from build123d import *

# Parameters (mm, degrees)
F1_DEPTH  = 8
F3_W      = 8
F3_H      = 8
F3_R      = 2.4
F4_DEPTH  = 1.7
F5_R      = 2.4
F6_DEPTH  = 1.7
F11_W     = 31.0510899872
F11_H     = 25.4
F12_DEPTH = 7.9248


with BuildPart() as f1:
    # F0 (on Front) → F1 (new body)
    with BuildSketch(Plane.XZ):
        Polygon((-2.4, 9.6), (-4, 9.6), (-4, 0), (4, 0), (4, 9.6), (2.4, 9.6), (2.4, 11.3), (-2.4, 11.3), align=None)
    extrude(amount=F1_DEPTH)

    # F3 (on plane+point) → F4 (cut, through all)
    with BuildSketch(Plane.XY.offset(11.3)):
        with Locations((0, -4)):
            Rectangle(F3_W, F3_H)
        with Locations((0, -4)):
            Circle(F3_R, mode=Mode.SUBTRACT)
    extrude(amount=-F4_DEPTH, mode=Mode.SUBTRACT)

    # F5 (on Top) → F6 (cut)
    with BuildSketch(Plane.XY):
        with Locations((0, -4)):
            Circle(F5_R)
    extrude(amount=F6_DEPTH, mode=Mode.SUBTRACT)

    # F8: F1 across plane


with BuildPart() as f1_1:
    add(f1.part)
    add(f1.part.mirror(Plane.YZ.offset(4)))

    # F9: F1 across face


with BuildPart() as f1_2:
    add(f1_1.part)
    add(f1_1.part.mirror(Plane(origin=(4, -8, 4.8), x_dir=(1, 0, 0), z_dir=(0, -1, 0))))

    # F10: F1 across face


with BuildPart() as f1_3:
    add(f1_2.part)
    add(f1_2.part.mirror(Plane(origin=(4, -16, 4.8), x_dir=(1, 0, 0), z_dir=(0, -1, 0))))

    # F11 (on Front) → F12 (cut)
    with BuildSketch(Plane.XZ):
        with Locations((3.3294046298, 0)):
            Rectangle(F11_W, F11_H)
    extrude(amount=F12_DEPTH, mode=Mode.SUBTRACT)


solid = f1_3.part
Could you check a few things on this model? Use its own coordinates, in mm. A direction names the side the tool comes from. Round coordinates to 2 decimals unless told otherwise and drop trailing zeros. Write each loop counter-clockwise with the first axis right and the second up, starting at its lowest first coordinate (ties: lowest second). Pieces come first, ordered by that corner, then holes. Notation, with made-up numbers: (-5.75, -16) - (26.25, -16) arc R24 cw to (26.25, -6) - close; hole circle Ø10 at (17, 79.5). An arc over 180 degrees is marked (long way). Put each result on its own line as item: value. Start each with the question number.
(1) I want a section at C-C, the plane y = -29.5. Please give me the cut outline in (x, z), plus the area to 3 significant figures.
(2) Will this pin go through, and if not, where does the flat tip stop? pin 1 (2 mm diameter, centred on x = 8, y = -11.5, fed in from -Z).
(3) For faces 1 (the flat face through (4, -20, 0)), 2 (the cylindrical face through (8.52, -22.343, 10.462)), 3 (the flat face through (8, -20, 1.7)), which set-ups out of +Z, -Z, +X, -X, +Y, -Y let a thin tool reach every point of the face, with its end or its side?
(4) Thinking about a two-plate mould opening in Y: for faces 4 (the flat face through (12, -20, 5)), 5 (the flat face through (8, -28, 1.7)), 6 (the flat face through (4, -7.925, 5)), 7 (the cylindrical face through (8.52, -22.343, 0.838)), which applies, released by +Y, released by -Y, zero draft, split by the parting line, or undercut?
(5) I need wall thicknesses on probe 1 along Y at (x, z) = (8, 0.6); probe 2 along X at (y, z) = (-28, 0.65); probe 3 along X at (y, z) = (-13.25, 1.5). Which ranges of each line are inside material? Lowest first, please.
(6) I want a section at B-B, the plane x = 0. Please give me the cut outline in (y, z), plus the area to 3 significant figures.
(7) I want a section at A-A, the plane z = 10. Please give me the cut outline in (x, y), plus the area to 3 significant figures.
Here are the results:
1. outline: (-4, 0) - (-1.87, 0) - (-1.87, 1.7) - (1.87, 1.7) - (1.87, 0) - (6.13, 0) - (6.13, 1.7) - (9.87, 1.7) - (9.87, 0) - (12, 0) - (12, 9.6) - (9.87, 9.6) - (9.87, 11.3) - (6.13, 11.3) - (6.13, 9.6) - (1.87, 9.6) - (1.87, 11.3) - (-1.87, 11.3) - (-1.87, 9.6) - (-4, 9.6) - close
1. area: 154 mm^2
2. pin 1: stops at z = 1.7
3. face 1: -Z, +X, -X, +Y, -Y
3. face 2: +Z
3. face 3: -Z
4. face 4: zero draft
4. face 5: undercut
4. face 6: released by +Y
4. face 7: undercut
5. probe 1: y = -32 to -30.4, -25.6 to -22.4, -17.6 to -14.4, -9.6 to -7.92
5. probe 2: x = -4 to -2.4, 2.4 to 5.6, 10.4 to 12
5. probe 3: x = -4 to -2.05, 2.05 to 5.95, 10.05 to 12
6. outline: (-32, 0) - (-30.4, 0) - (-30.4, 1.7) - (-25.6, 1.7) - (-25.6, 0) - (-22.4, 0) - (-22.4, 1.7) - (-17.6, 1.7) - (-17.6, 0) - (-14.4, 0) - (-14.4, 1.7) - (-9.6, 1.7) - (-9.6, 0) - (-7.92, 0) - (-7.92, 9.6) - (-9.6, 9.6) - (-9.6, 11.3) - (-14.4, 11.3) - (-14.4, 9.6) - (-17.6, 9.6) - (-17.6, 11.3) - (-22.4, 11.3) - (-22.4, 9.6) - (-25.6, 9.6) - (-25.6, 11.3) - (-30.4, 11.3) - (-30.4, 9.6) - (-32, 9.6) - close
6. area: 231 mm^2
7. outline: circle Ø4.8 at (0, -28); circle Ø4.8 at (0, -20); circle Ø4.8 at (0, -12); circle Ø4.8 at (8, -28); circle Ø4.8 at (8, -20); circle Ø4.8 at (8, -12)
7. area: 109 mm^2
